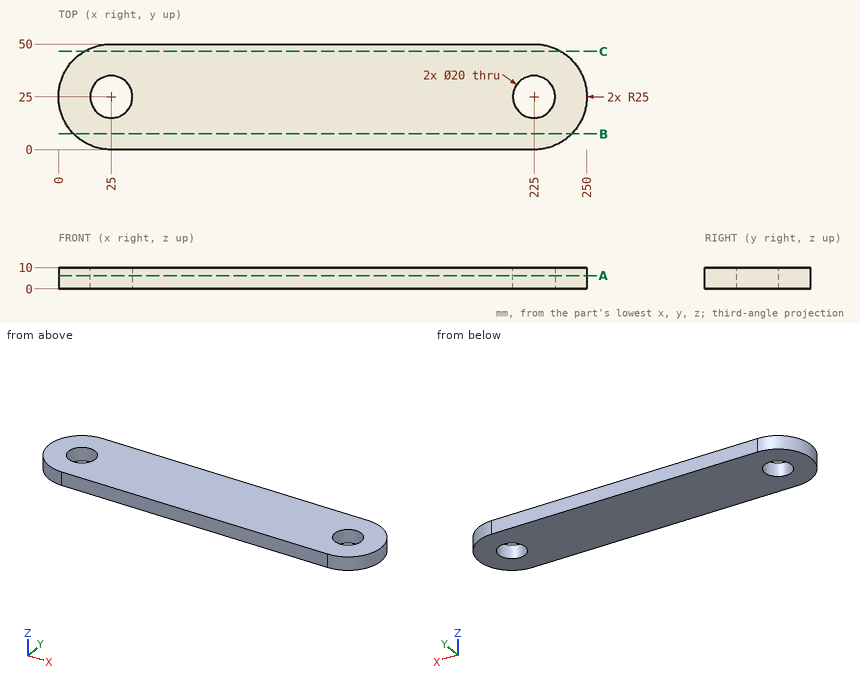
Design review of the part shown in the three views and the two pictorial views. Dimensions are in mm from the part's minimum x, y and z. Round coordinates to 2 decimals unless told otherwise and drop trailing zeros. Loops run counter-clockwise (first coordinate to the right, second up) from the corner with the lowest first, then second, coordinate; pieces in that order, holes last. Notation, with made-up numbers: (49, 87) -> (100, 87) arc R24 ccw to (100, 99) -> close; hole circle Ø8 at (54, 86). An arc over 180 degrees is marked (long way). Use one line per item in the form item = value. Start each with the question number.
Q1. Wall thickness on line 1 along Y through (x, z) = (25, 6); line 2 along X through (y, z) = (29.5, 5); line 3 along X through (y, z) = (38, 1.75): over which ranges is each line inside the solid? List them lowest first. Write a range as [from, to].
Q2. We need section C-C on y = 46.5. Give the boundary of the cut face in (x, z).
Q3. We need section A-A on z = 6.25. Give the boundary of the cut face in (x, y), then the cut area to 3 significant figures.
Q4. We need section B-B on y = 7.5. Give the boundary of the cut face in (x, z).
Q5. For pin 1 Ø4 at (y, z) = (5.5, 3.5) entering from +X; pin 2 Ø1 at (y, z) = (22, 2.5) entering from -X; pin 3 Ø1.5 at (y, z) = (17, 3.5) entering from -X, all flat-tipped, find the tip position at first contact; note any pin that passes through.
Calculated:
q1.line_1 = [0, 15], [35, 50]
q1.line_2 = [0.41, 16.07], [33.93, 216.07], [233.93, 249.59]
q1.line_3 = [3.65, 246.35]
q2.outline = (12.24, 0) -> (237.76, 0) -> (237.76, 10) -> (12.24, 10) -> close
q3.outline = (25, 0) -> (225, 0) arc R25 ccw to (225, 50) -> (25, 50) arc R25 ccw to start; hole circle Ø20 at (25, 25); hole circle Ø20 at (225, 25)
q3.area = 11,300 mm²
q4.outline = (7.15, 0) -> (242.85, 0) -> (242.85, 10) -> (7.15, 10) -> close
q5.pin_1 = 242.85
q5.pin_2 = 0.13
q5.pin_3 = 1.07
